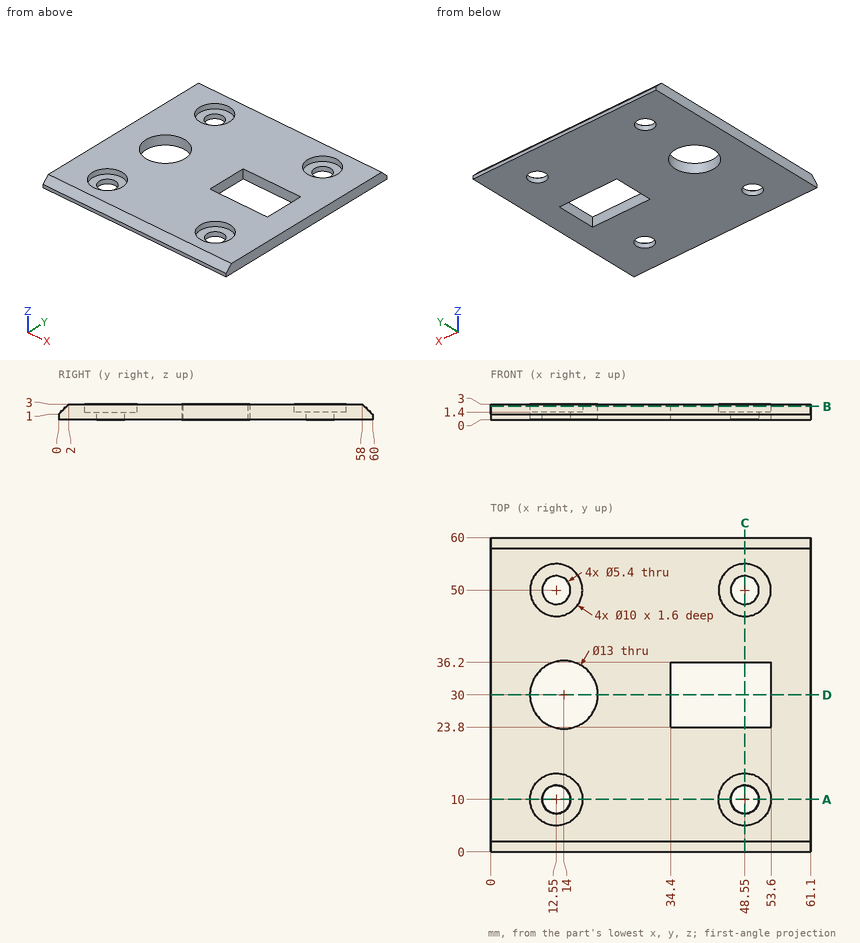
For this review, use the dimensioned drawing (mm, ordinates from the lowest corner) and the shaded views. Coordinates: 2 decimals unless noted, no trailing zeros. Write each loop counter-clockwise with the first axis right and the second up, starting at its lowest first coordinate (ties: lowest second). Pieces come first, ordered by that corner, then holes. Notation, with made-up numbers: (31.5, 32.5) - (60.5, 32.5) arc R24 ccw to (60.5, 61.5) - close; hole circle Ø7 at (46, 24). An arc over 180 degrees is marked (long way). One line per item, written item: value.
1) Add section A-A (y = 10). State the section outline as (x, z) points, plus the area to 3 significant figures.
Answer sheet:
outline: (0, 0) - (9.85, 0) - (9.85, 1.4) - (7.55, 1.4) - (7.55, 3) - (0, 3) - close; (15.25, 0) - (45.85, 0) - (45.85, 1.4) - (43.55, 1.4) - (43.55, 3) - (17.55, 3) - (17.55, 1.4) - (15.25, 1.4) - close; (51.25, 0) - (61.1, 0) - (61.1, 3) - (53.55, 3) - (53.55, 1.4) - (51.25, 1.4) - close
area: 136 mm2
2) Add section C-C (x = 48.55). State the section outline as (y, z) points.
Answer sheet:
outline: (0, 0) - (7.3, 0) - (7.3, 1.4) - (5, 1.4) - (5, 3) - (2, 3) - (0, 1) - close; (12.7, 0) - (23.8, 0) - (23.8, 3) - (15, 3) - (15, 1.4) - (12.7, 1.4) - close; (36.2, 0) - (47.3, 0) - (47.3, 1.4) - (45, 1.4) - (45, 3) - (36.2, 3) - close; (52.7, 0) - (60, 0) - (60, 1) - (58, 3) - (55, 3) - (55, 1.4) - (52.7, 1.4) - close
3) Add section D-D (y = 30). State the section outline as (x, z) points, plus the area to 3 significant figures.
Answer sheet:
outline: (0, 0) - (7.5, 0) - (7.5, 3) - (0, 3) - close; (20.5, 0) - (34.4, 0) - (34.4, 3) - (20.5, 3) - close; (53.6, 0) - (61.1, 0) - (61.1, 3) - (53.6, 3) - close
area: 86.7 mm2
4) Add section B-B (z = 2.55). State the section outline as (x, y) points, plus the area to 3 significant figures.
Answer sheet:
outline: (0, 1.55) - (61.1, 1.55) - (61.1, 58.45) - (0, 58.45) - close; hole circle Ø13 at (14, 30); hole circle Ø10 at (12.55, 10); hole circle Ø10 at (12.55, 50); hole (34.4, 23.8) - (53.6, 23.8) - (53.6, 36.2) - (34.4, 36.2) - close; hole circle Ø10 at (48.55, 10); hole circle Ø10 at (48.55, 50)
area: 2,790 mm2
5) To check wall thickness, follow probe 1 along Y at (x, z) = (48.5, 0.75); probe 2 along X at (y, z) = (24, 2.4); probe 3 along X at (y, z) = (33, 0.85). State the ranges of each line that lie inside material, in increasing order.
Answer sheet:
probe 1: y = 0 to 7.3, 12.7 to 23.8, 36.2 to 47.3, 52.7 to 60
probe 2: x = 0 to 11.5, 16.5 to 34.4, 53.6 to 61.1
probe 3: x = 0 to 8.23, 19.77 to 34.4, 53.6 to 61.1
6) Insertion check: pin 1 (3 mm diameter, centred on x = 50, y = 10.5, fed in from +Z). The pin has a flat end and moves straight along its axis. Give the tip position at first contact, or say it passes through.
Answer sheet:
pin 1: stops at z = 1.4
